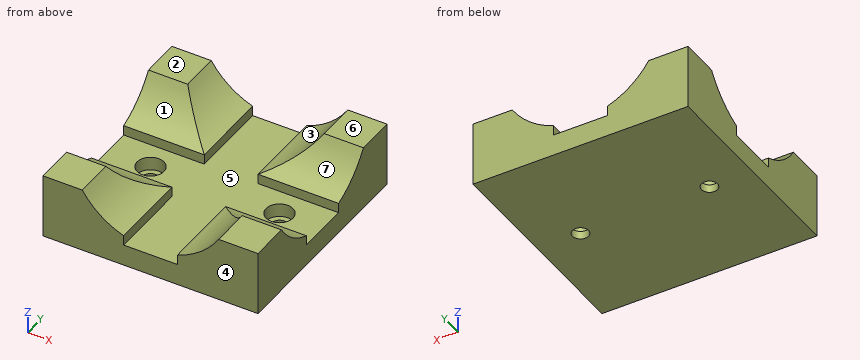
```python
from build123d import *

# Parameters (mm, degrees)
SKETCH1_W           = 40
SKETCH1_H           = 40
BOSS_EXTRUDE1_DEPTH = 12
CUT_EXTRUDE1_DEPTH  = 40
SKETCH3_R           = 2.5
CUT_EXTRUDE3_DEPTH  = 40
SKETCH3_5_R         = 2.5
SKETCH3_5_R_2       = 1.5
BOSS_EXTRUDE3_DEPTH = 1.5
CIRPATTERN3_COUNT   = 2
CIRPATTERN3_ANGLE   = 90


with BuildPart() as part:
    # Sketch1 → Boss-Extrude1 (new body)
    with BuildSketch(Plane.XY):
        with Locations((20, 20)):
            Rectangle(SKETCH1_W, SKETCH1_H)
    extrude(amount=BOSS_EXTRUDE1_DEPTH)

    # Sketch2 → Cut-Extrude1 (cut)
    with BuildSketch(Plane(origin=(40, 0, 0), x_dir=(0, 0, -1), z_dir=(1, 0, 0))):
        with BuildLine():
            Line((-5, 25), (-4, 25))
            Line((-4, 25), (-4, 15))
            Line((-4, 15), (-5, 15))
            Line((-5, 15), (-5.857864376, 15))
            ThreePointArc((-5.857864376, 15), (-35, 20), (-5.857864376, 25))
            Line((-5.857864376, 25), (-5, 25))
        make_face()
    cut_extrude1 = extrude(amount=-CUT_EXTRUDE1_DEPTH, mode=Mode.SUBTRACT)

    # Sketch3 → Cut-Extrude3 (cut)
    with BuildSketch(Plane(origin=(0, 0, 0), x_dir=(-1, 0, 0), z_dir=(0, 0, -1))):
        with Locations((-32, 20)):
            Circle(SKETCH3_R)
        with Locations((-8, 20)):
            Circle(SKETCH3_R)
    extrude(amount=-CUT_EXTRUDE3_DEPTH, mode=Mode.SUBTRACT)

    # Sketch3<5> → Boss-Extrude3 (add)
    # profile 1 of 2: a face of its own
    with BuildSketch(Plane(origin=(0, 0, 0), x_dir=(-1, 0, 0), z_dir=(0, 0, -1))):
        with Locations((-32, 20)):
            Circle(SKETCH3_5_R)
        with Locations((-32, 20)):
            Circle(SKETCH3_5_R_2, mode=Mode.SUBTRACT)
    # profile 2 of 2: a face of its own
    with BuildSketch(Plane(origin=(0, 0, 0), x_dir=(-1, 0, 0), z_dir=(0, 0, -1))):
        with Locations((-8, 20)):
            Circle(SKETCH3_5_R)
        with Locations((-8, 20)):
            Circle(SKETCH3_5_R_2, mode=Mode.SUBTRACT)
    extrude(amount=-BOSS_EXTRUDE3_DEPTH)

    # CirPattern3: Cut-Extrude1 ×2 about axis
    cirpattern3_axis = Axis((20, 20, 4), (0, 0, 1))
    for i in range(1, CIRPATTERN3_COUNT):
        add(cut_extrude1.rotate(cirpattern3_axis, i * CIRPATTERN3_ANGLE / (CIRPATTERN3_COUNT - 1)), mode=Mode.SUBTRACT)


solid = part.part
```
Geometry: final body of the model. Coordinates: model frame, mm. Face numbers are marked on the shaded views. A direction names the side the tool comes from. Coordinates: 2 decimals unless noted, no trailing zeros. Write each loop counter-clockwise with the first axis right and the second up, starting at its lowest first coordinate (ties: lowest second). Pieces come first, ordered by that corner, then holes. Notation, with made-up numbers: M -26.5,85 L -15.5,85 A26 cw -15.5,100 Z; hole C 68.25,41.25 d9. An arc over 180 degrees is marked long. Use CSV: the item, a comma, the result in double quotes. Start each with the question number.
1. Mould query, pull axis Y, two halves, no side actions, for the marked faces 4, 5, 6 and 7. Classes: pulls with the +Y half, pulls with the -Y half, needs draft (parallel to the pull), parting line crosses it, or undercut.
2. Reachability of the marked faces 1, 2 and 3 from +Z, -Z, +X, -X, +Y, -Y: full face, straight path, thin tool, end or side. Return the list, or none.
3. Cut plane C-C on y = 36. Return the cut outline in (x, z).
4. Cut plane B-B on x = 8. Return the cut outline in (y, z).
5. First-contact query: P1, Ø2.5, axis at x = 8, y = 19, coming from the +Z side. Flat tip, straight axial feed; report the tip coordinate or a pass-through.
6. Cut plane A-A on y = 20. Return the cut outline in (x, z).
7. Cut plane D-D on z = 7.5. Return the cut outline in (x, y), plus the area to 3 significant figures.
8. Ray query, probe 1 along X at (y, z) = (8, 5); probe 2 along Y at (x, z) = (32, 3.3); probe 3 along Y at (x, z) = (32, 0.65). Return the intervals inside material, ascending.
Entries:
1,face 4,"pulls with the -Y half"
1,face 5,"undercut"
1,face 6,"needs draft"
1,face 7,"undercut"
2,face 1,"+Z, +X, -X"
2,face 2,"+Z, +X, -X, +Y, -Y"
2,face 3,"+Z, +Y, -Y"
3,outline,"M 0,0 L 40,0 L 40,12 L 32.69,12 A15 cw 25,5.86 L 25,4 L 15,4 L 15,5.86 A15 cw 7.31,12 L 0,12 Z"
4,outline,"M 0,0 L 18.5,0 L 18.5,1.5 L 17.5,1.5 L 17.5,4 L 15,4 L 15,5.86 A15 cw 8,11 L 0,11 Z; M 21.5,0 L 40,0 L 40,11 L 32,11 A15 cw 25,5.86 L 25,4 L 22.5,4 L 22.5,1.5 L 21.5,1.5 Z"
5,P1,"z = 1.5"
6,outline,"M 0,0 L 6.5,0 L 6.5,1.5 L 5.5,1.5 L 5.5,4 L 0,4 Z; M 9.5,0 L 30.5,0 L 30.5,1.5 L 29.5,1.5 L 29.5,4 L 10.5,4 L 10.5,1.5 L 9.5,1.5 Z; M 33.5,0 L 40,0 L 40,4 L 34.5,4 L 34.5,1.5 L 33.5,1.5 Z"
7,outline,"M 0,0 L 11.71,0 L 11.71,11.71 L 0,11.71 Z; M 0,28.29 L 11.71,28.29 L 11.71,40 L 0,40 Z; M 28.29,0 L 40,0 L 40,11.71 L 28.29,11.71 Z; M 28.29,28.29 L 40,28.29 L 40,40 L 28.29,40 Z"
7,area,"548 mm²"
8,probe 1,"0 to 15, 25 to 40"
8,probe 2,"0 to 17.5, 22.5 to 40"
8,probe 3,"0 to 18.5, 21.5 to 40"
